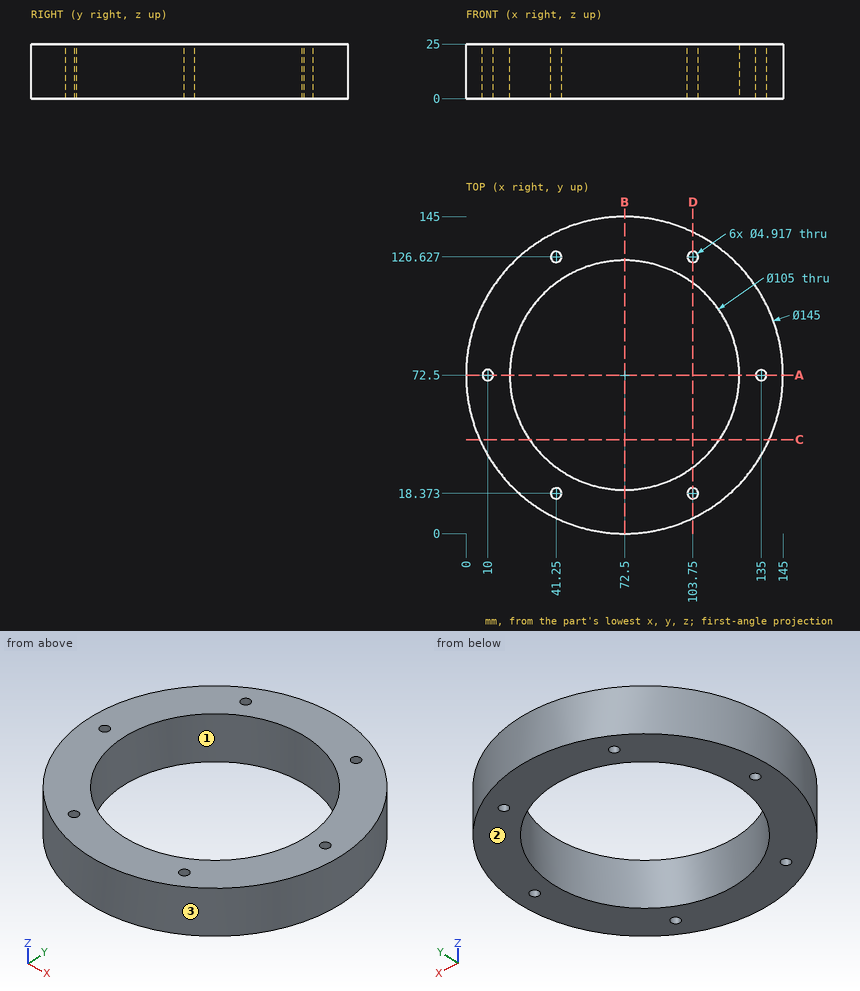
Can you work these out from the drawing? Everything is in mm from the part's minimum corner. Coordinates: 2 decimals unless noted, no trailing zeros. Loops run counter-clockwise (first coordinate to the right, second up) from the corner with the lowest first, then second, coordinate; pieces in that order, holes last.
1) Thinking about a two-plate mould opening in X: for the marked faces 1, 2 and 3, which applies, released by +X, released by -X, zero draft, split by the parting line, or undercut?
Reported:
face 1: undercut
face 2: zero draft
face 3: split by the parting line
2) Imagine slicing it at A-A (y = 72.5). List the corners of the cut face in (x, z) for me.
Reported:
outline: (0, 0) - (7.54, 0) - (7.54, 25) - (0, 25) - close; (12.46, 0) - (20, 0) - (20, 25) - (12.46, 25) - close; (125, 0) - (132.54, 0) - (132.54, 25) - (125, 25) - close; (137.46, 0) - (145, 0) - (145, 25) - (137.46, 25) - close
3) Please list where these lines run through material, in increasing order: line 1 along Y through (x, z) = (72.5, 8.75); line 2 along X through (y, z) = (73, 21.75); line 3 along X through (y, z) = (99, 6.5) (1 decimal).
Reported:
line 1: y = 0 to 20, 125 to 145
line 2: x = 0 to 7.59, 12.41 to 20, 125 to 132.59, 137.41 to 145
line 3: x = 5 to 27.2, 117.8 to 140
4) Imagine slicing it at C-C (y = 43). List the corners of the cut face in (x, z) for me, and give its area (3 significant figures).
Reported:
outline: (6.27, 0) - (29.07, 0) - (29.07, 25) - (6.27, 25) - close; (115.93, 0) - (138.73, 0) - (138.73, 25) - (115.93, 25) - close
area: 1,140 mm2
5) Imagine slicing it at B-B (x = 72.5). List the corners of the cut face in (y, z) for me, and give its area (3 significant figures).
Reported:
outline: (0, 0) - (20, 0) - (20, 25) - (0, 25) - close; (125, 0) - (145, 0) - (145, 25) - (125, 25) - close
area: 1,000 mm2
6) Will these pins go through, and if not, where does the flat tip stop? pin 1 Ø5 at (x, z) = (17, 22) entering from -Y; pin 2 Ø1.5 at (x, z) = (28.5, 9) entering from +Y; pin 3 Ø1.5 at (x, z) = (118, 4.5) entering from -Y.
Reported:
pin 1: stops at y = 23.03
pin 2: stops at y = 130.69
pin 3: stops at y = 15.46
7) Imagine slicing it at D-D (x = 103.75). List the corners of the cut face in (y, z) for me (1 decimal).
Reported:
outline: (7.1, 0) - (15.9, 0) - (15.9, 25) - (7.1, 25) - close; (20.8, 0) - (30.3, 0) - (30.3, 25) - (20.8, 25) - close; (114.7, 0) - (124.2, 0) - (124.2, 25) - (114.7, 25) - close; (129.1, 0) - (137.9, 0) - (137.9, 25) - (129.1, 25) - close
